```python
from build123d import *

# Parameters (mm, degrees)
F0_W     = 54
F0_H     = 30
F0_R     = 1.5
F0_R_2   = 3.25
F1_DEPTH = 20
F3_R     = 2.5
F4_DEPTH = 16
F6_R     = 4.45
F7_DEPTH = 8
F5_R     = 3.25
F8_DEPTH = 8


with BuildPart() as f1:
    # F0 (on Front) → F1 (new body)
    with BuildSketch(Plane.XZ):
        with Locations((27, 15)):
            Rectangle(F0_W, F0_H)
        with Locations((47, 13.5)):
            Circle(F0_R, mode=Mode.SUBTRACT)
        with Locations((7, 16.5)):
            Circle(F0_R, mode=Mode.SUBTRACT)
        with Locations((25, 15)):
            Circle(F0_R_2, mode=Mode.SUBTRACT)
        with Locations((36, 15)):
            Circle(F0_R_2, mode=Mode.SUBTRACT)
    extrude(amount=F1_DEPTH)

    # F3 (on face) → F4 (cut)
    with BuildSketch(Plane(origin=(0, 0, 0), x_dir=(1, 0, 0), z_dir=(0, 0, -1))):
        with Locations((36, 10)):
            Circle(F3_R)
    extrude(amount=-F4_DEPTH, mode=Mode.SUBTRACT)

    # F6 (on face) → F7 (cut)
    with BuildSketch(Plane(origin=(0, 0, 0), x_dir=(-1, 0, 0), z_dir=(0, 1, 0))):
        with Locations((-25, 15)):
            Circle(F6_R)
    extrude(amount=-F7_DEPTH, mode=Mode.SUBTRACT)

    # F5 (on face) → F8 (join)
    with BuildSketch(Plane(origin=(0, 0, 0), x_dir=(-1, 0, 0), z_dir=(0, 1, 0))):
        with Locations((-36, 15)):
            Circle(F5_R)
    extrude(amount=-F8_DEPTH)


solid = f1.part
```
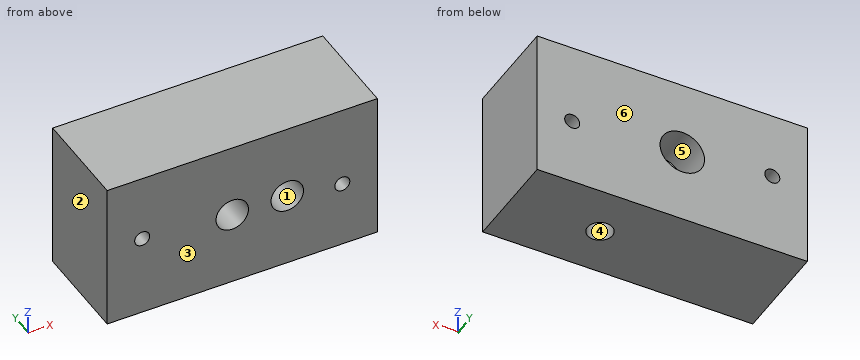
The listing builds one solid part. Answer for the finished solid, in the listing's coordinates (mm). Face numbers are marked on the shaded views. A direction names the side the tool comes from. Round coordinates to 2 decimals unless told otherwise and drop trailing zeros. Loops run counter-clockwise (first coordinate to the right, second up) from the corner with the lowest first, then second, coordinate; pieces in that order, holes last.
1) Consider line 1 (Z direction, x = 47, y = -15.5); line 2 (X direction, y = -10, z = 8.5); line 3 (Z direction, x = 25, y = -2.75). Determine where each line is inside the solid, lowest interval first.
Outcome:
line 1: z = 0 to 12, 15 to 30
line 2: x = 0 to 33.5, 38.5 to 54
line 3: z = 0 to 10.55, 19.45 to 30
2) A cutting plane is placed at D-D on y = -16.75. Determine the outline of the cut face in (x, z), plus the area to 3 significant figures.
Outcome:
outline: (0, 0) - (54, 0) - (54, 30) - (0, 30) - close; hole circle Ø3 at (7, 16.5); hole circle Ø6.5 at (25, 15); hole circle Ø6.5 at (36, 15); hole circle Ø3 at (47, 13.5)
area: 1,540 mm2
3) A cutting plane is placed at B-B on x = 36. Determine the outline of the cut face in (y, z).
Outcome:
outline: (-20, 0) - (-12.5, 0) - (-12.5, 11.75) - (-20, 11.75) - close; (-20, 18.25) - (-8, 18.25) - (-8, 11.75) - (-7.5, 11.75) - (-7.5, 0) - (0, 0) - (0, 30) - (-20, 30) - close
4) For the marked faces 4, 5 and 6, determine the directions among +Z, -Z, +X, -X, +Y, -Y from which every point of the face is accessible in a straight line to the end or side of a thin tool.
Outcome:
face 4: -Z
face 5: +Y
face 6: +Z, -Z, +X, -X, +Y
5) A cutting plane is placed at A-A on y = -5.25. Determine the outline of the cut face in (x, z), plus the area to 3 significant figures.
Outcome:
outline: (0, 0) - (54, 0) - (54, 30) - (0, 30) - close; hole circle Ø3 at (7, 16.5); hole circle Ø8.9 at (25, 15); hole circle Ø3 at (47, 13.5)
area: 1,540 mm2
6) Given P1, Ø3.5, axis at x = 47, z = 13.5, coming from the +Y side; P2, Ø3, axis at x = 37.5, z = 15.5, coming from the -Y side, each flat-ended and moving along its own axis, determine where each tip first touches the part or whether it passes through.
Outcome:
P1: stops at y = 0
P2: stops at y = -8
7) For a pull along X with two mould halves and no side action, classify the marked faces 1, 2 and 3 as released by +X, released by -X, zero draft, split by the parting line, or undercut.
Outcome:
face 1: undercut
face 2: released by -X
face 3: zero draft
8) A cutting plane is placed at C-C on z = 16.5. Determine the outline of the cut face in (x, y).
Outcome:
outline: (0, -20) - (5.5, -20) - (5.5, 0) - (0, 0) - close; (8.5, -20) - (22.12, -20) - (22.12, -8) - (20.81, -8) - (20.81, 0) - (8.5, 0) - close; (27.88, -20) - (33.12, -20) - (33.12, -8) - (38.88, -8) - (38.88, -20) - (54, -20) - (54, 0) - (29.19, 0) - (29.19, -8) - (27.88, -8) - close
